Verification items for the finished model (mm, model axes). Face numbers are marked on the shaded views. A direction names the side the tool comes from. Give positions to 0.01 mm unless a question says otherwise; leave off trailing zeros. Order: outer loops, then holes, each group sorted by start corner. A loop starts at its lowest first (then second) coordinate and runs counter-clockwise, first axis right, second up. Notation, with made-up numbers: (37.5, 46.5) - (79.5, 46.5) arc R15 ccw to (79.5, 57.5) - close; hole circle Ø4 at (-5.5, 47). An arc over 180 degrees is marked (long way). Answer as a JSON object with one key per item and string values. Group by question number.
(1) Section check A-A (y = 4.5). Record the boundary of the cut face in (x, z), then the cut area to 3 significant figures.
(2) Section check C-C (y = -12.7). Record the boundary of the cut face in (x, z).
(3) Thickness scan on line 1 (Z direction, x = 36, y = 5.5); line 2 (X direction, y = 2.5, z = 27). Record the ranges inside material, lowest first.
(4) Section check B-B (z = 24). Record the boundary of the cut face in (x, y), then the cut area to 3 significant figures.
(5) Section check D-D (x = 22). Record the boundary of the cut face in (y, z).
(6) Depth check by flat-ended pin: pin 1 Ø8 at (y, z) = (-3, 13.5) entering from +X; pin 2 Ø6 at (x, z) = (10.5, 5) entering from +Y; pin 3 Ø6 at (x, y) = (20, 13.5) entering from +Z. Enter the tip coordinate at first touch or a pass-through.
(7) Access from +Z, -Z, +X, -X, +Y, -Y to the whole of each face (thin tool, end or side, straight path). Record for the marked faces 1 and 2.
```python
from build123d import *

# Parameters (mm, degrees)
EXTRUDE_THIN1_START          = -19.05
EXTRUDE_THIN1_DEPTH          = 38.1
SKETCH4_R                    = 2.0828
EXTRUDE3_DEPTH               = 57.145492036
SKETCH5_R                    = 2.0828
CUT_EXTRUDE1_DEPTH           = 2.54
CUT_EXTRUDE1_DRAFT           = 41
CUT_EXTRUDE1_PROFILE_2_DEPTH = 2.54
CUT_EXTRUDE1_PROFILE_2_DRAFT = 41
CUT_EXTRUDE1_PROFILE_3_DEPTH = 2.54
CUT_EXTRUDE1_PROFILE_3_DRAFT = 41
MIRROR1_COPY_1_SKETCH_R      = 2.0828
MIRROR1_COPY_1_DEPTH         = 2.54
MIRROR1_COPY_1_DRAFT         = 41
MIRROR1_COPY_2_SKETCH_R      = 2.0828
MIRROR1_COPY_2_DEPTH         = 2.54
MIRROR1_COPY_2_DRAFT         = 41
MIRROR1_COPY_3_SKETCH_R      = 2.0828
MIRROR1_COPY_3_DEPTH         = 2.54
MIRROR1_COPY_3_DRAFT         = 41
MIRROR1_COPY_4_SKETCH_R      = 2.0828
MIRROR1_COPY_4_DEPTH         = 2.54
MIRROR1_COPY_4_DRAFT         = 41
MIRROR1_COPY_5_SKETCH_R      = 2.0828
MIRROR1_COPY_5_DEPTH         = 2.54
MIRROR1_COPY_5_DRAFT         = 41


# Read off the part's stored shape, not the designer's step: Extrude-Thin1
with BuildPart() as part:
    # Extrude-Thin1 outline → Extrude-Thin1 (new body)
    with BuildSketch(Plane(origin=(0, 0, 0), x_dir=(1, 0, 0), z_dir=(0, 1, 0)).offset(EXTRUDE_THIN1_START)):
        with BuildLine():
            Line((2.286, -1.524), (38.1, -1.524))
            Line((38.1, -1.524), (38.1, 0))
            Line((38.1, 0), (2.286, 0))
            ThreePointArc((2.286, 0), (0.669553898, -0.669553898), (0, -2.286))
            Line((0, -2.286), (0, -38.1))
            Line((0, -38.1), (1.524, -38.1))
            Line((1.524, -38.1), (1.524, -2.286))
            ThreePointArc((1.524, -2.286), (1.747184633, -1.747184633), (2.286, -1.524))
        make_face()
    extrude(amount=EXTRUDE_THIN1_DEPTH)

    # Sketch4 → Extrude3 (cut, through all)
    with BuildSketch(Plane(origin=(1.524, 0, 0), x_dir=(0, 0, -1), z_dir=(1, 0, 0))):
        with Locations((-28.575, 0)):
            Circle(SKETCH4_R)
        with Locations((-14.2748, 12.7)):
            Circle(SKETCH4_R)
        with Locations((-14.2748, -12.7)):
            Circle(SKETCH4_R)
    extrude3 = extrude(amount=-EXTRUDE3_DEPTH, mode=Mode.SUBTRACT)


with BuildPart() as cut_extrude1_tool:
    # Sketch5 → Cut-Extrude1 (with draft: the straight prism first)
    with BuildSketch(Plane.ZY):
        with Locations((14.2748, -12.7)):
            Circle(SKETCH5_R)
    extrude(amount=-CUT_EXTRUDE1_DEPTH)
    # Cut-Extrude1: the draft: its side faces are tilted about the plane it starts from
    cut_extrude1_sides = [cut_extrude1_tool.faces().sort_by_distance(p)[0] for p in [
        (1.27, -12.7, 12.192),
    ]]
    draft(cut_extrude1_sides, Plane.ZY, CUT_EXTRUDE1_DRAFT)


with BuildPart() as part_1:
    add(part.part)

    # Cut-Extrude1: cut by cut_extrude1_tool
    add(cut_extrude1_tool.part, mode=Mode.SUBTRACT)


with BuildPart() as cut_extrude1_profile_2_tool:
    # Sketch5 → Cut-Extrude1 profile 2 (with draft: the straight prism first)
    with BuildSketch(Plane.ZY):
        with Locations((14.2748, 12.7)):
            Circle(SKETCH5_R)
    extrude(amount=-CUT_EXTRUDE1_PROFILE_2_DEPTH)
    # Cut-Extrude1 profile 2: the draft: its side faces are tilted about the plane it starts from
    cut_extrude1_profile_2_sides = [cut_extrude1_profile_2_tool.faces().sort_by_distance(p)[0] for p in [
        (1.27, 12.7, 12.192),
    ]]
    draft(cut_extrude1_profile_2_sides, Plane.ZY, CUT_EXTRUDE1_PROFILE_2_DRAFT)


with BuildPart() as part_2:
    add(part_1.part)

    # Cut-Extrude1 profile 2: cut by cut_extrude1_profile_2_tool
    add(cut_extrude1_profile_2_tool.part, mode=Mode.SUBTRACT)


with BuildPart() as cut_extrude1_profile_3_tool:
    # Sketch5 → Cut-Extrude1 profile 3 (with draft: the straight prism first)
    with BuildSketch(Plane.ZY):
        with Locations((28.575, 0)):
            Circle(SKETCH5_R)
    extrude(amount=-CUT_EXTRUDE1_PROFILE_3_DEPTH)
    # Cut-Extrude1 profile 3: the draft: its side faces are tilted about the plane it starts from
    cut_extrude1_profile_3_sides = [cut_extrude1_profile_3_tool.faces().sort_by_distance(p)[0] for p in [
        (1.27, 0, 26.4922),
    ]]
    draft(cut_extrude1_profile_3_sides, Plane.ZY, CUT_EXTRUDE1_PROFILE_3_DRAFT)


with BuildPart() as part_3:
    add(part_2.part)

    # Cut-Extrude1 profile 3: cut by cut_extrude1_profile_3_tool
    add(cut_extrude1_profile_3_tool.part, mode=Mode.SUBTRACT)

    # Mirror1: Extrude3 across plane
    add(extrude3.mirror(Plane(origin=(0, 0, 0), x_dir=(0.7071067811865465, 0, 0.7071067811865486), z_dir=(-0.7071067811865488, 0, 0.7071067811865464))), mode=Mode.SUBTRACT)


with BuildPart() as mirror1_copy_1_tool:
    # Mirror1 copy 1 sketch → Mirror1 copy 1 (with draft: the straight prism first)
    with BuildSketch(Plane(origin=(0, 0, 0), x_dir=(1, 0, 0), z_dir=(0, 0, -1))):
        with Locations((14.2748, 12.7)):
            Circle(MIRROR1_COPY_1_SKETCH_R)
    extrude(amount=-MIRROR1_COPY_1_DEPTH)
    # Mirror1 copy 1: the draft: its side faces are tilted about the plane it starts from
    mirror1_copy_1_sides = [mirror1_copy_1_tool.faces().sort_by_distance(p)[0] for p in [
        (12.192, -12.7, 1.27),
    ]]
    draft(mirror1_copy_1_sides, Plane(origin=(0, 0, 0), x_dir=(1, 0, 0), z_dir=(0, 0, -1)), MIRROR1_COPY_1_DRAFT)


with BuildPart() as part_4:
    add(part_3.part)

    # Mirror1 copy 1: cut by mirror1_copy_1_tool
    add(mirror1_copy_1_tool.part, mode=Mode.SUBTRACT)


with BuildPart() as mirror1_copy_2_tool:
    # Mirror1 copy 2 sketch → Mirror1 copy 2 (with draft: the straight prism first)
    with BuildSketch(Plane(origin=(0, 0, 0), x_dir=(1, 0, 0), z_dir=(0, 0, -1))):
        with Locations((14.2748, -12.7)):
            Circle(MIRROR1_COPY_2_SKETCH_R)
    extrude(amount=-MIRROR1_COPY_2_DEPTH)
    # Mirror1 copy 2: the draft: its side faces are tilted about the plane it starts from
    mirror1_copy_2_sides = [mirror1_copy_2_tool.faces().sort_by_distance(p)[0] for p in [
        (12.192, 12.7, 1.27),
    ]]
    draft(mirror1_copy_2_sides, Plane(origin=(0, 0, 0), x_dir=(1, 0, 0), z_dir=(0, 0, -1)), MIRROR1_COPY_2_DRAFT)


with BuildPart() as part_5:
    add(part_4.part)

    # Mirror1 copy 2: cut by mirror1_copy_2_tool
    add(mirror1_copy_2_tool.part, mode=Mode.SUBTRACT)


with BuildPart() as mirror1_copy_3_tool:
    # Mirror1 copy 3 sketch → Mirror1 copy 3 (with draft: the straight prism first)
    with BuildSketch(Plane(origin=(0, 0, 0), x_dir=(1, 0, 0), z_dir=(0, 0, -1))):
        with Locations((28.575, 0)):
            Circle(MIRROR1_COPY_3_SKETCH_R)
    extrude(amount=-MIRROR1_COPY_3_DEPTH)
    # Mirror1 copy 3: the draft: its side faces are tilted about the plane it starts from
    mirror1_copy_3_sides = [mirror1_copy_3_tool.faces().sort_by_distance(p)[0] for p in [
        (26.4922, 0, 1.27),
    ]]
    draft(mirror1_copy_3_sides, Plane(origin=(0, 0, 0), x_dir=(1, 0, 0), z_dir=(0, 0, -1)), MIRROR1_COPY_3_DRAFT)


with BuildPart() as part_6:
    add(part_5.part)

    # Mirror1 copy 3: cut by mirror1_copy_3_tool
    add(mirror1_copy_3_tool.part, mode=Mode.SUBTRACT)


with BuildPart() as mirror1_copy_4_tool:
    # Mirror1 copy 4 sketch → Mirror1 copy 4 (with draft: the straight prism first)
    with BuildSketch(Plane(origin=(0, 0, 0), x_dir=(1, 0, 0), z_dir=(0, 0, -1))):
        with Locations((14.2748, -12.7)):
            Circle(MIRROR1_COPY_4_SKETCH_R)
    extrude(amount=-MIRROR1_COPY_4_DEPTH)
    # Mirror1 copy 4: the draft: its side faces are tilted about the plane it starts from
    mirror1_copy_4_sides = [mirror1_copy_4_tool.faces().sort_by_distance(p)[0] for p in [
        (12.192, 12.7, 1.27),
    ]]
    draft(mirror1_copy_4_sides, Plane(origin=(0, 0, 0), x_dir=(1, 0, 0), z_dir=(0, 0, -1)), MIRROR1_COPY_4_DRAFT)


with BuildPart() as part_7:
    add(part_6.part)

    # Mirror1 copy 4: cut by mirror1_copy_4_tool
    add(mirror1_copy_4_tool.part, mode=Mode.SUBTRACT)


with BuildPart() as mirror1_copy_5_tool:
    # Mirror1 copy 5 sketch → Mirror1 copy 5 (with draft: the straight prism first)
    with BuildSketch(Plane(origin=(0, 0, 0), x_dir=(1, 0, 0), z_dir=(0, 0, -1))):
        with Locations((28.575, 0)):
            Circle(MIRROR1_COPY_5_SKETCH_R)
    extrude(amount=-MIRROR1_COPY_5_DEPTH)
    # Mirror1 copy 5: the draft: its side faces are tilted about the plane it starts from
    mirror1_copy_5_sides = [mirror1_copy_5_tool.faces().sort_by_distance(p)[0] for p in [
        (26.4922, 0, 1.27),
    ]]
    draft(mirror1_copy_5_sides, Plane(origin=(0, 0, 0), x_dir=(1, 0, 0), z_dir=(0, 0, -1)), MIRROR1_COPY_5_DRAFT)


with BuildPart() as part_8:
    add(part_7.part)

    # Mirror1 copy 5: cut by mirror1_copy_5_tool
    add(mirror1_copy_5_tool.part, mode=Mode.SUBTRACT)


solid = part_8.part
```
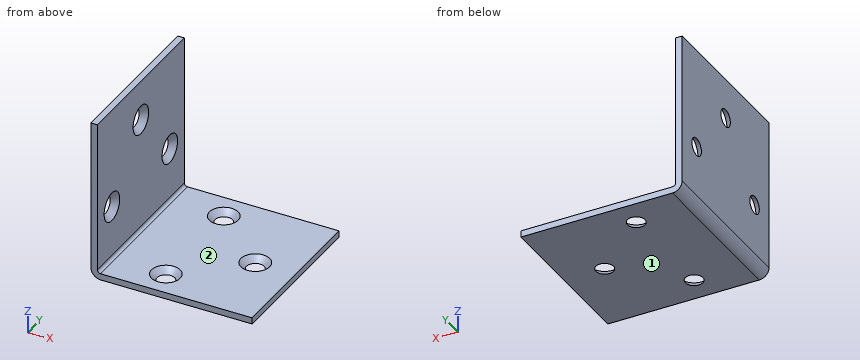
Solutions:
{
 "1": {"outline": "(0, 2.29) arc R2.29 ccw to (2.29, 0) - (38.1, 0) - (38.1, 1.52) - (2.29, 1.52) arc R0.76 cw to (1.52, 2.29) - (1.52, 38.1) - (0, 38.1) - close", "area": "113 mm2"},
 "2": {"outline": "(0, 2.29) arc R2.29 ccw to (2.29, 0) - (12.19, 0) - (10.87, 1.52) - (2.29, 1.52) arc R0.76 cw to (1.52, 2.29) - (1.52, 10.87) - (0, 12.19) - close; (0, 16.36) - (1.52, 17.68) - (1.52, 38.1) - (0, 38.1) - close; (16.36, 0) - (38.1, 0) - (38.1, 1.52) - (17.68, 1.52) - close"},
 "3": {"line 1": "z = 0 to 1.52", "line 2": "x = 0 to 1"},
 "4": {"outline": "(0, -19.05) - (1.52, -19.05) - (1.52, 19.05) - (0, 19.05) - close", "area": "58.1 mm2"},
 "5": {"outline": "(-19.05, 0) - (19.05, 0) - (19.05, 1.52) - (-19.05, 1.52) - close"},
 "6": {"pin 1": "stops at x = 1.52", "pin 2": "passes through", "pin 3": "stops at z = 1.52"},
 "7": {"face 1": "-Z, +X, -X, +Y, -Y", "face 2": "+Z, +X, +Y, -Y"}
}
